For this review, use the dimensioned drawing (mm, ordinates from the lowest corner) and the shaded views. Round coordinates to 2 decimals unless told otherwise and drop trailing zeros. Write each question's results on one line, items separated by ' | '. Start each with the question number.
(1) Take a section at A-A, the plane z = 2. Give the number of separate pieces and of enclosed holes in the cut face, plus the area to 3 significant figures.
(2) For L1, parallel to X at y = 3.75, z = 0.5; L2, parallel to X at y = 2.75, z = 2.25 (1 decimal); L3, parallel to X at y = 1.75, z = 3.5 (1 decimal), list the stretches that pass through material, from the lowest coordinate up. Write a range as from..to.
(3) Insertion check: pin 1 Ø3 at (x, y) = (5.5, 2) entering from +Z (3 decimals); pin 2 Ø1 at (y, z) = (2.5, 5.5) entering from -X. Each pin has a flat end and moves straight along its axis. Give the tip position at first contact, or say it passes through.
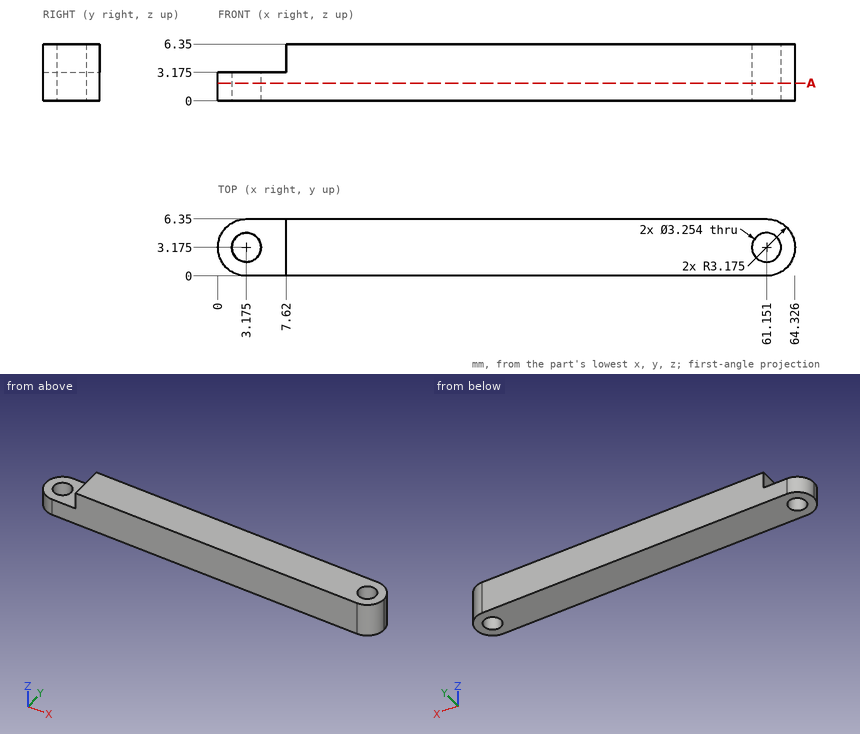
Results below:
1) separate pieces: 1 | enclosed holes: 2 | area: 383 mm^2
2) L1: x = 0.05..1.65, 4.7..59.63, 62.67..64.27 | L2: x = 0..1.6, 4.7..59.6, 62.7..64.3 | L3: x = 7.6..60.4, 61.9..64
3) pin 1: stops at z = 3.175 | pin 2: stops at x = 7.62
